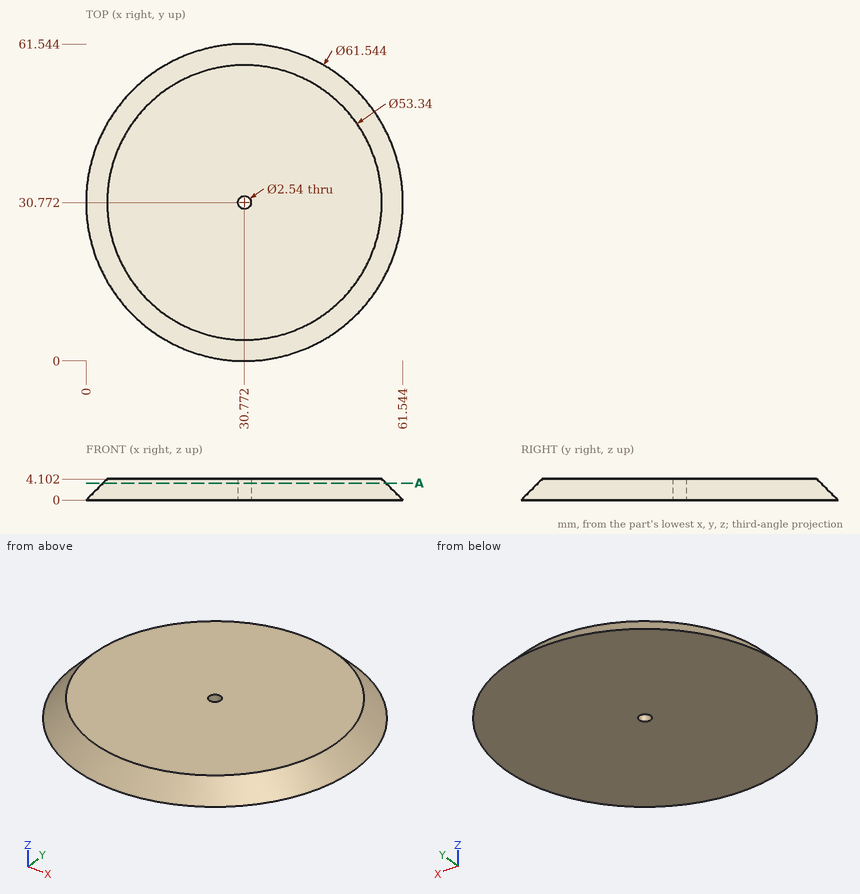
Job drawing, mm, ordinate dimensions from the low corner. One solid piece. Give positions to 0.01 mm unless a question says otherwise; leave off trailing zeros. Order: outer loops, then holes, each group sorted by start corner. A loop starts at its lowest first (then second) coordinate and runs counter-clockwise, first axis right, second up. Notation, with made-up numbers: M 9.25,-33 L 45.25,-33 A35 ccw 45.25,6 Z; hole C 78,43.5 d1. An arc over 180 degrees is marked long. Put each result on its own line as item: value. Start each with the question number.
(1) Drill centre lines: L1, parallel to X at y = 16.5, z = 0.8 (1 decimal); L2, parallel to Y at x = 43, z = 0.4 (1 decimal); L3, parallel to Y at x = 50, z = 1.6 (1 decimal). Where is each one in solid material? Low to high. Write a range as [from, to].
(2) Band-saw the part on A-A on z = 3.3. Give the cut face in (x, y), then the cut area to 3 significant figures.
(3) Pin check, flat tips, straight feed: pin 1 Ø2 at (x, y) = (47.5, 6.5) entering from +Z (1 decimal); pin 2 Ø1.5 at (x, z) = (34, 1) entering from -Y. Stop position of each tip, or through.
Results below:
1. L1: x = [4.4, 57.1]
1. L2: y = [3, 58.6]
1. L3: y = [8.8, 52.7]
2. outline: C 30.77,30.77 d54.94; hole C 30.77,30.77 d2.54
2. area: 2,370 mm2
3. pin 1: stops at z = 2.3
3. pin 2: stops at y = 0.42
